Here's how the part is built. I have some questions about the finished solid (model axes, mm). Face numbers are marked on the shaded views. A direction names the side the tool comes from. Round coordinates to 2 decimals unless told otherwise and drop trailing zeros. Write each loop counter-clockwise with the first axis right and the second up, starting at its lowest first coordinate (ties: lowest second). Pieces come first, ordered by that corner, then holes. Notation, with made-up numbers: (64, 76) - (94, 76) arc R32 cw to (94, 103) - close; hole circle Ø9 at (74, -5). An arc over 180 degrees is marked (long way). Write item = value, one per line. Start each with the question number.
Item 1: If I drill on line 1 along Z through (x, y) = (6.5, 9.5); line 2 along X through (y, z) = (9.25, -6.5); line 3 along Z through (x, y) = (2.75, 3), over which ranges is the centre line in solid material (lowest first)? Write a range as [from, to].
Item 2: For P1, Ø1.3, axis at y = 3, z = -6.5, coming from the -X side, with a flat end and sliding along its axis, tell me the tip position at first contact or that it passes through.
Item 3: Thinking about a two-plate mould opening in X: for the marked faces 1, 2 and 3, which applies, pulls with the +X half, pulls with the -X half, needs draft (parallel to the pull), parting line crosses it, or undercut?
Item 4: If we section it at D-D (y = 2.25): Please give me the cut outline in (x, z).
Item 5: Which directions (+Z, -Z, +X, -X, +Y, -Y) give clear straight access to the entire face, cutting with the end or side of a thin tool? Please do the marked faces 4, 5, 6, 7 and 8.
Item 6: If we section it at B-B (z = -7.25): Please give me the cut outline in (x, y).
Item 7: If we section it at A-A (x = 8.75): Please give me the cut outline in (y, z).
Item 8: If we section it at C-C (y = 5.5): Please give me the cut outline in (x, z) (3 decimals), and give its area (3 significant figures).
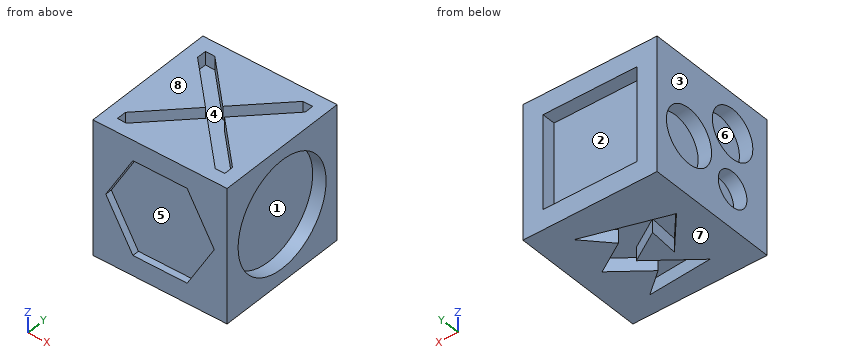
```python
from build123d import *

# Parameters (mm, degrees)
SKETCH2_W           = 10
SKETCH2_H           = 10
BOSS_EXTRUDE1_DEPTH = 10
CUT_EXTRUDE1_DEPTH  = 1
SKETCH4_R           = 4
CUT_EXTRUDE2_DEPTH  = 1
SKETCH5_W           = 7
SKETCH5_H           = 7
CUT_EXTRUDE3_DEPTH  = 1
CUT_EXTRUDE4_DEPTH  = 1
SKETCH7_R           = 1.303792798
SKETCH7_R_2         = 2.05363311
SKETCH7_R_3         = 1.840686576
CUT_EXTRUDE5_DEPTH  = 1
CUT_EXTRUDE13_DEPTH = 0.5


with BuildPart() as part:
    # Sketch2 → Boss-Extrude1 (new body)
    with BuildSketch(Plane(origin=(0, 0, 0), x_dir=(1, 0, 0), z_dir=(0, 1, 0))):
        with Locations((5, 5)):
            Rectangle(SKETCH2_W, SKETCH2_H)
    extrude(amount=BOSS_EXTRUDE1_DEPTH)

    # Sketch3 → Cut-Extrude1 (cut)
    with BuildSketch(Plane.XY):
        Polygon((8.305584857, 0.987308362), (9.012691638, 0.987308362), (9.012691638, 1.694415143), (5.707106781, 5), (9.012691638, 8.305584857), (9.012691638, 8.987308362), (8.280201581, 8.987308362), (5, 5.707106781), (1.719798419, 8.987308362), (1.012691638, 8.987308362), (1.012691638, 8.280201581), (4.292893219, 5), (1.012691638, 1.719798419), (1.012691638, 0.987308362), (1.694415143, 0.987308362), (5, 4.292893219), align=None)
    extrude(amount=-CUT_EXTRUDE1_DEPTH, mode=Mode.SUBTRACT)

    # Sketch4 → Cut-Extrude2 (cut)
    with BuildSketch(Plane(origin=(10, 0, 0), x_dir=(0, 0, -1), z_dir=(1, 0, 0))):
        with Locations((5, 5)):
            Circle(SKETCH4_R)
    extrude(amount=-CUT_EXTRUDE2_DEPTH, mode=Mode.SUBTRACT)

    # Sketch5 → Cut-Extrude3 (cut)
    with BuildSketch(Plane(origin=(0, 10, 0), x_dir=(1, 0, 0), z_dir=(0, 1, 0))):
        with Locations((5, 5)):
            Rectangle(SKETCH5_W, SKETCH5_H)
    extrude(amount=-CUT_EXTRUDE3_DEPTH, mode=Mode.SUBTRACT)

    # Sketch6 → Cut-Extrude4 (cut)
    with BuildSketch(Plane(origin=(0, 0, -10), x_dir=(-1, 0, 0), z_dir=(0, 0, -1))):
        Polygon((-7.691273898, 8.169929887), (-1.596078599, 6.292074313), (-3.945946393, 3.612705427), (-3.762984072, 5.82237163), (-6.145851296, 4.385481263), (-2.771012496, 1.810947861), (-7.54308372, 1.463168774), (-5.754546035, 2.887207167), (-8.32224735, 4.846006741), (-5.924161107, 6.292074313), align=None)
    extrude(amount=-CUT_EXTRUDE4_DEPTH, mode=Mode.SUBTRACT)

    # Sketch7 → Cut-Extrude5 (cut)
    with BuildSketch(Plane.ZY):
        with Locations((-7.072203837, 3.137345215)):
            Circle(SKETCH7_R)
        with Locations((-5.589634204, 7.102221042)):
            Circle(SKETCH7_R_2)
        with Locations((-2.980104129, 3.137345215)):
            Circle(SKETCH7_R_3)
    extrude(amount=-CUT_EXTRUDE5_DEPTH, mode=Mode.SUBTRACT)

    # Sketch9 → Cut-Extrude13 (cut)
    with BuildSketch(Plane(origin=(0, 0, 0), x_dir=(-1, 0, 0), z_dir=(0, -1, 0))):
        Polygon((-9.041451884, 5), (-7.020725942, 1.5), (-2.979274058, 1.5), (-0.958548116, 5), (-2.979274058, 8.5), (-7.020725942, 8.5), align=None)
    extrude(amount=-CUT_EXTRUDE13_DEPTH, mode=Mode.SUBTRACT)


solid = part.part
```
Reply:
q1.line_1 = [-10, -8.5], [-1.5, 0]
q1.line_2 = [0, 1.5], [8.5, 10]
q1.line_3 = [-10, -1]
q2.P1 = 1
q3.face_1 = pulls with the +X half
q3.face_2 = undercut
q3.face_3 = pulls with the -X half
q4.outline = (0, -10) - (3.35, -10) - (3.35, -9) - (6.55, -9) - (6.55, -10) - (10, -10) - (10, -7.9) - (9, -7.9) - (9, -2.1) - (10, -2.1) - (10, 0) - (8.46, 0) - (8.46, -1) - (7.04, -1) - (7.04, 0) - (2.96, 0) - (2.96, -1) - (1.54, -1) - (1.54, 0) - (0, 0) - (0, -1.37) - (1, -1.37) - (1, -4.59) - (0, -4.59) - (0, -6.12) - (1, -6.12) - (1, -8.03) - (0, -8.03) - close
q5.face_4 = +Z
q5.face_5 = -Y
q5.face_6 = -X
q5.face_7 = -Z, +X, -X, +Y, -Y
q5.face_8 = +Z, +X, -X, +Y, -Y
q6.outline = (0, 0) - (2.26, 0) - (2.26, 0.5) - (7.74, 0.5) - (7.74, 0) - (10, 0) - (10, 1.69) - (9, 1.69) - (9, 8.31) - (10, 8.31) - (10, 10) - (8.5, 10) - (8.5, 9) - (1.5, 9) - (1.5, 10) - (0, 10) - (0, 8.31) - (1, 8.31) - (1, 5.89) - (0, 5.89) - (0, 4.43) - (1, 4.43) - (1, 1.85) - (0, 1.85) - close
q7.outline = (0, -10) - (10, -10) - (10, 0) - (8.99, 0) - (8.99, -1) - (8.04, -1) - (8.04, 0) - (1.96, 0) - (1.96, -1) - (0.99, -1) - (0.99, 0) - (0, 0) - (0, -4.5) - (0.5, -4.5) - (0.5, -5.5) - (0, -5.5) - close
q8.outline = (0, -10) - (2.291, -10) - (2.291, -9) - (3.79, -9) - (3.79, -10) - (4.298, -10) - (4.298, -9) - (7.238, -9) - (7.238, -10) - (10, -10) - (10, -8.969) - (9, -8.969) - (9, -1.031) - (10, -1.031) - (10, 0) - (6.207, 0) - (6.207, -1) - (3.793, -1) - (3.793, 0) - (0, 0) - (0, -4.305) - (1, -4.305) - (1, -6.874) - (0, -6.874) - close
q8.area = 82.6 mm2
